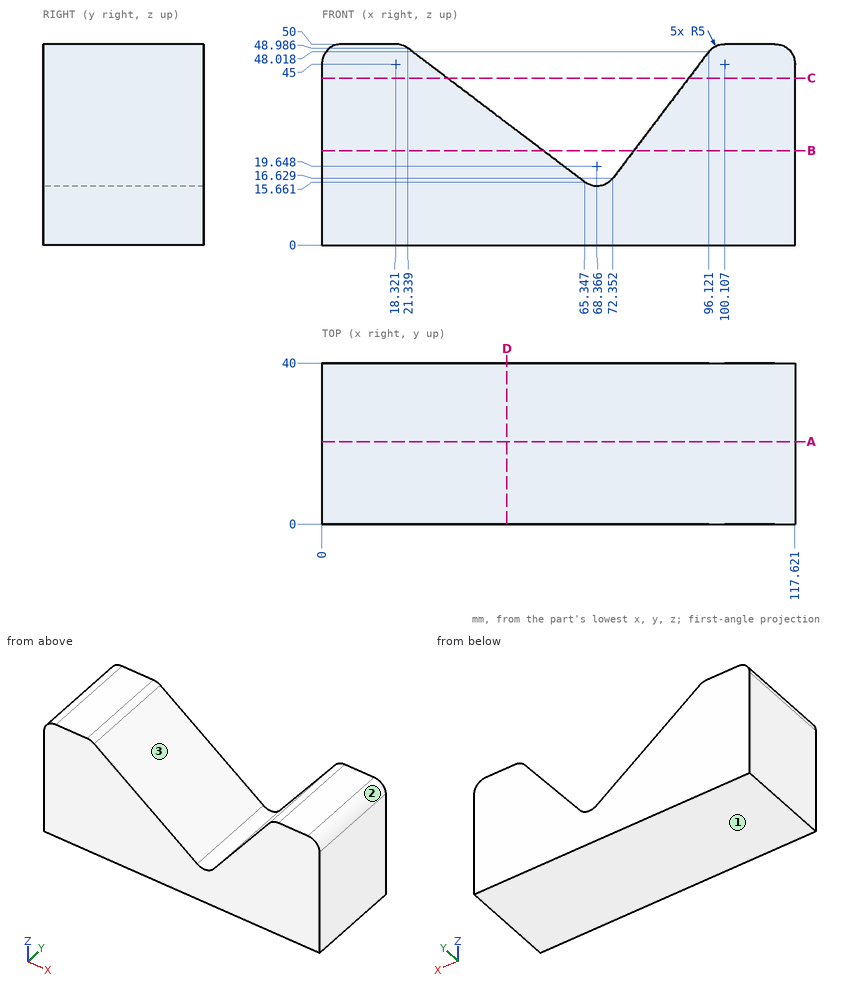
Here's the drawing with two shaded views (mm, measured from the low corner). I have some questions. Round coordinates to 2 decimals unless told otherwise and drop trailing zeros. Order: outer loops, then holes, each group sorted by start corner. A loop starts at its lowest first (then second) coordinate and runs counter-clockwise, first axis right, second up. Notation, with made-up numbers: (-22, 50.5) -> (-13, 50.5) arc R30 ccw to (-13, 73.5) -> close; hole circle Ø1 at (39, 68). An arc over 180 degrees is marked (long way). Write each question's results on one line, items separated by ' | '. Start each with the question number.
Item 1: If we section it at D-D, the plane x = 46: Write out the boundary of the cut face in (y, z), then the cut area to 3 significant figures.
Item 2: If we section it at B-B, the plane z = 23.5: Write out the boundary of the cut face in (x, y) (1 decimal).
Item 3: If we section it at A-A, the plane y = 20.5: Write out the boundary of the cut face in (x, z) (1 decimal).
Item 4: Will this pin go through, and if not, where does the flat tip stop? pin 1 (3 mm diameter, centred on x = 88, y = 33.5, fed in from +Z) (1 decimal).
Item 5: Please list where these lines run through material, in increasing order: L1, parallel to X at y = 28.5, z = 36.5 (1 decimal); L2, parallel to X at y = 9, z = 20 (1 decimal); L3, parallel to Z at x = 22, y = 19 (1 decimal).
Item 6: If we section it at C-C, the plane z = 41.5: Write out the boundary of the cut face in (x, y) (1 decimal).
Item 7: Thinking about a two-plate mould opening in X: for the marked faces 1, 2 and 3, which applies, +X half, -X half, draft (parallel to the pull), parting line (faces both ways), or undercut?
Results:
1) outline: (0, 0) -> (40, 0) -> (40, 30.31) -> (0, 30.31) -> close | area: 1,210 mm2
2) outline: (0, 0) -> (55, 0) -> (55, 40) -> (0, 40) -> close; (77.6, 0) -> (117.6, 0) -> (117.6, 40) -> (77.6, 40) -> close
3) outline: (0, 0) -> (117.6, 0) -> (117.6, 45) arc R5 ccw to (112.6, 50) -> (100.1, 50) arc R5 ccw to (96.1, 48) -> (72.4, 16.6) arc R5 cw to (65.3, 15.7) -> (21.3, 49) arc R5 ccw to (18.3, 50) -> (5, 50) arc R5 ccw to (0, 45) -> close
4) pin 1: stops at z = 39.3
5) L1: x = 0 to 37.8, 87.4 to 117.6 | L2: x = 0 to 59.6, 74.9 to 117.6 | L3: z = 0 to 48.5
6) outline: (0, 0) -> (31.2, 0) -> (31.2, 40) -> (0, 40) -> close; (91.2, 0) -> (117.6, 0) -> (117.6, 40) -> (91.2, 40) -> close
7) face 1: draft | face 2: +X half | face 3: undercut
